from build123d import *

# Parameters (mm, degrees)
RESSALTO_EXTRUS_O1_DEPTH = 5
ESBO_O2_R                = 40
ESBO_O2_R_2              = 30
EXTRUS_O_FINA1_DEPTH     = 18
ESBO_O7_R                = 18
CORTE_EXTRUS_O2_DEPTH    = 1.5
CORTE_EXTRUS_O9_DEPTH    = 128.5


with BuildPart() as part:
    # Esboço1 → Ressalto-extrusão1 (new body)
    with BuildSketch(Plane(origin=(0, 0, 0), x_dir=(1, 0, 0), z_dir=(0, 1, 0))):
        with BuildLine():
            Line((-35.169337018, 43.205430296), (14.830662982, 43.205430296))
            ThreePointArc((14.830662982, 43.205430296), (32.508332512, 35.883099826), (39.830662982, 18.205430296))
            Line((39.830662982, 18.205430296), (39.830662982, -31.794569704))
            ThreePointArc((39.830662982, -31.794569704), (32.508332512, -49.472239233), (14.830662982, -56.794569704))
            Line((14.830662982, -56.794569704), (-35.169337018, -56.794569704))
            ThreePointArc((-35.169337018, -56.794569704), (-52.847006547, -49.472239233), (-60.169337018, -31.794569704))
            Line((-60.169337018, -31.794569704), (-60.169337018, 18.205430296))
            ThreePointArc((-60.169337018, 18.205430296), (-52.847006547, 35.883099826), (-35.169337018, 43.205430296))
        make_face()
    extrude(amount=RESSALTO_EXTRUS_O1_DEPTH)

    # Esboço2 → Extrusão-Fina1 (add)
    with BuildSketch(Plane(origin=(0, 5, 0), x_dir=(1, 0, 0), z_dir=(0, 1, 0))):
        with Locations((-10.169337018, -6.794569704)):
            Circle(ESBO_O2_R)
        with Locations((-10.169337018, -6.794569704)):
            Circle(ESBO_O2_R_2, mode=Mode.SUBTRACT)
    extrude(amount=EXTRUS_O_FINA1_DEPTH)

    # Esboço7 → Corte-extrusão2 (cut)
    with BuildSketch(Plane(origin=(0, 5, 0), x_dir=(1, 0, 0), z_dir=(0, 1, 0))):
        with Locations(Location((-10.169337018, -6.794569704, 0), (0, 0, 270))):
            Circle(ESBO_O7_R)
    extrude(amount=-CORTE_EXTRUS_O2_DEPTH, mode=Mode.SUBTRACT)

    # Esboço16 → Corte-extrusão9 (cut)
    with BuildSketch(Plane(origin=(0, 0, -43.205430296), x_dir=(-1, 0, 0), z_dir=(0, 0, -1))):
        Polygon((-29.830662982, 14), (64.710384206, 14), (64.710384206, 40.871723048), (-29.830662982, 40.871723048), (-67.520218161, 40.871723048), (-67.520218161, 14), align=None)
    extrude(amount=-CORTE_EXTRUS_O9_DEPTH, mode=Mode.SUBTRACT)


solid = part.part
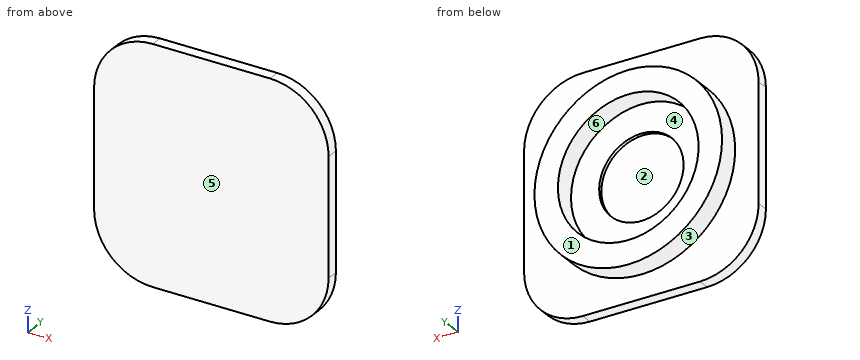
Here's how the part is built. I have some questions about the finished solid (model axes, mm). Face numbers are marked on the shaded views. A direction names the side the tool comes from. Round coordinates to 2 decimals unless told otherwise and drop trailing zeros. Order: outer loops, then holes, each group sorted by start corner. A loop starts at its lowest first (then second) coordinate and runs counter-clockwise, first axis right, second up. Notation, with made-up numbers: M 4,63 L 59,63 A12 ccw 59,69 Z; hole C -8,10 d6. An arc over 180 degrees is marked long. Return JSON: item names as keys, results as strings. Group by question number.
1. If we section it at D-D on z = -30.5: List the corners of the cut face in (x, y) for me.
2. On a 3-axis mill with a long thin cutter (end or side, diameter ignored), from which of +Z, -Z, +X, -X, +Y, -Y can I reach the whole of each face in a straight line? I mean the marked faces 1 and 2. Say none if no direction works.
3. If we mould it in two halves opening along X, with no side actions, what happens to the marked faces 3, 4, 5 and 6? For each: pulls with the +X half, pulls with the -X half, needs draft (parallel to the pull), parting line crosses it, or undercut.
4. Please list where these lines run through material, in increasing order: probe 1 along Y at (x, z) = (-27, -37.5); probe 2 along X at (y, z) = (6.5, -13); probe 3 along X at (y, z) = (5.25, -10).
5. If we section it at C-C on z = -13.5: List the corners of the cut face in (x, y) for me.
6. I'm going to push flat-ended pins straight in: pin 1 Ø10 at (x, z) = (-18, 13.5) entering from +Y; pin 2 Ø2 at (x, y) = (-36, 11.5) entering from +Z; pin 3 Ø1.5 at (x, y) = (22, 5) entering from -Z. Where does each tip first touch, or does it pass through?
7. If we section it at B-B on x = -16: List the corners of the cut face in (y, z) for me.
8. If we section it at A-A on y = 1.75: List the corners of the cut face in (x, z) for me.
Reply:
{
 "1": {"outline": "M -56.94,0 L 36.6,0 L 36.6,5 L 4.29,5 L 4.29,14 L -24.63,14 L -24.63,5 L -56.94,5 Z"},
 "2": {"face 1": "+Z, -Z, +X, -X, +Y", "face 2": "+Y"},
 "3": {"face 3": "parting line crosses it", "face 4": "undercut", "face 5": "needs draft", "face 6": "undercut"},
 "4": {"probe 1": "0 to 5", "probe 2": "-44.93 to -32.71, 12.37 to 24.59", "probe 3": "-46.47 to -35.03, 14.69 to 26.13"},
 "5": {"outline": "M -60.17,0 L 39.83,0 L 39.83,5 L 24.3,5 L 24.3,14 L 11.92,14 L 11.92,5 L -32.26,5 L -32.26,14 L -44.64,14 L -44.64,5 L -60.17,5 Z"},
 "6": {"pin 1": "y = 3.5", "pin 2": "z = 38.15", "pin 3": "z = -42.37"},
 "7": {"outline": "M 0,-43.21 L 5,-43.21 L 5,-32.78 L 14,-32.78 L 14,-22.63 L 5,-22.63 L 5,-10.23 L 3.5,-10.23 L 3.5,23.82 L 5,23.82 L 5,36.22 L 14,36.22 L 14,46.37 L 5,46.37 L 5,56.79 L 0,56.79 Z"},
 "8": {"outline": "M -60.17,-18.21 A25 ccw -35.17,-43.21 L 14.83,-43.21 A25 ccw 39.83,-18.21 L 39.83,31.79 A25 ccw 14.83,56.79 L -35.17,56.79 A25 ccw -60.17,31.79 Z"}
}
